from build123d import *

# Parameters (mm, degrees)
F1_DEPTH = 6.35
F2_W     = 4.6636089683
F2_H     = 11.6590159014
F2_H_2   = 4.0806564502
F2_W_2   = 10.2016367018
F2_W_3   = 10.7845924795
F2_H_3   = 15.7396723516
F3_DEPTH = 6.35
F4_W     = 5.2465572953
F4_H     = 11.0760659445
F4_H_2   = 4.0806552861
F4_W_2   = 11.076066643
F4_W_3   = 10.4931145906
F4_H_3   = 15.1567212306
F5_DEPTH = 6.35


with BuildPart() as f1:
    # F0 (on Top) → F1 (new body)
    with BuildSketch(Plane.XY):
        Polygon((72.8688538074, 28.418853879), (-66.7478665709, 28.418853879), (-66.7478665709, -67.4765557051), (-11.9504919276, -67.4765557051), (-11.9504919276, -25.212623179), (15.7396737486, -25.212623179), (15.7396737486, -67.4765557051), (72.8688538074, -67.4765557051), align=None)
        Polygon((-50.1337721944, 0), (-50.1337721944, 15.0109836832), (-37.7460662276, 15.0109836832), (-25.3583602607, 15.0109836832), (-25.3583602607, 0), (-25.3583602607, -15.0109836832), (-37.7460662276, -15.0109836832), (-50.1337721944, -15.0109836832), align=None, mode=Mode.SUBTRACT)
        Polygon((35.2685265243, 0), (35.2685265243, 15.0109836832), (46.7818062752, 15.0109836832), (58.2950860262, 15.0109836832), (58.2950860262, 0), (58.2950860262, -15.0109836832), (46.7818062752, -15.0109836832), (35.2685265243, -15.0109836832), align=None, mode=Mode.SUBTRACT)
        Polygon((0, 76.5122994781), (-66.7478665709, 28.418853879), (72.8688538074, 28.418853879), align=None)
    extrude(amount=F1_DEPTH)

    # F2 (on Top) → F3 (join)
    with BuildSketch(Plane.XY):
        with Locations((46.0531152785, 9.7644259222)):
            Rectangle(F2_W, F2_H)
        with Locations((46.0531152785, 1.8945897464)):
            Rectangle(F2_W, F2_H_2)
        with Locations((38.6204924434, 1.8945897464)):
            Rectangle(F2_W_2, F2_H_2)
        with Locations((53.7772160023, 1.8945897464)):
            Rectangle(F2_W_3, F2_H_2)
        with Locations((46.0531152785, -8.0155746546)):
            Rectangle(F2_W, F2_H_3)
    extrude(amount=F3_DEPTH)

    # F4 (on Top) → F5 (join)
    with BuildSketch(Plane.XY):
        with Locations((-38.1832793355, 9.1814756161)):
            Rectangle(F4_W, F4_H)
        with Locations((-38.1832793355, 1.6031150008)):
            Rectangle(F4_W, F4_H_2)
        with Locations((-46.3445913047, 1.6031150008)):
            Rectangle(F4_W_2, F4_H_2)
        with Locations((-30.3134433925, 1.6031150008)):
            Rectangle(F4_W_3, F4_H_2)
        with Locations((-38.1832793355, -8.0155732576)):
            Rectangle(F4_W, F4_H_3)
    extrude(amount=F5_DEPTH)


solid = f1.part
Source: CAD feature listing. Evaluate the final solid. Frame: model axes, mm. A direction names the side the tool comes from. Round coordinates to 2 decimals unless told otherwise and drop trailing zeros. Order: outer loops, then holes, each group sorted by start corner. A loop starts at its lowest first (then second) coordinate and runs counter-clockwise, first axis right, second up. Notation, with made-up numbers: (61, 19) -> (98, 19) arc R32 ccw to (98, 50) -> close; hole circle Ø5 at (52, 28.5). An arc over 180 degrees is marked (long way). Answer as CSV lines item,"result".
Item 1: Section C-C, the plane y = -12. Return loops of the section in (x, z), plus the area to 3 significant figures.
A:
outline,"(-66.75, 0) -> (-50.13, 0) -> (-50.13, 6.35) -> (-66.75, 6.35) -> close; (-40.81, 0) -> (-35.56, 0) -> (-35.56, 6.35) -> (-40.81, 6.35) -> close; (-25.36, 0) -> (35.27, 0) -> (35.27, 6.35) -> (-25.36, 6.35) -> close; (43.72, 0) -> (48.38, 0) -> (48.38, 6.35) -> (43.72, 6.35) -> close; (58.3, 0) -> (72.87, 0) -> (72.87, 6.35) -> (58.3, 6.35) -> close"
area,"646 mm²"
Item 2: Section B-B, the plane x = 55.5. Return loops of the section in (y, z).
A:
outline,"(-67.48, 0) -> (-15.01, 0) -> (-15.01, 6.35) -> (-67.48, 6.35) -> close; (-0.15, 0) -> (3.93, 0) -> (3.93, 6.35) -> (-0.15, 6.35) -> close; (15.01, 0) -> (39.88, 0) -> (39.88, 6.35) -> (15.01, 6.35) -> close"
Item 3: Pin query (flat end, axial travel): pin 1 Ø1 at (y, z) = (43.5, 3) entering from -X; pin 2 Ø1 at (x, z) = (50.5, 4) entering from +Y. Return the tip coordinate at first contact, or that it passes through.
A:
pin 1,"x = -46.51"
pin 2,"y = 43.51"
Item 4: Reachability of faces 1 (the face through (39, 3.935, 3)), 2 (the face through (72.869, -20, 3)) from +Z, -Z, +X, -X, +Y, -Y: full face, straight path, thin tool, end or side. Return the list, or none.
A:
face 1,"+Z, -Z"
face 2,"+Z, -Z, +X, +Y, -Y"
Item 5: Line query: L1, parallel to X at y = 9, z = 6; L2, parallel to X at y = -37.5, z = 2; L3, parallel to Y at x = 41, z = 2.5. Output: solid intervals per line, ascending.
A:
L1,"-66.75 to -50.13, -40.81 to -35.56, -25.36 to 35.27, 43.72 to 48.38, 58.3 to 72.87"
L2,"-66.75 to -11.95, 15.74 to 72.87"
L3,"-67.48 to -15.01, -0.15 to 3.93, 15.01 to 49.45"
Item 6: Section A-A, the plane y = -27.5. Return loops of the section in (x, z), plus the area to 3 significant figures.
A:
outline,"(-66.75, 0) -> (-11.95, 0) -> (-11.95, 6.35) -> (-66.75, 6.35) -> close; (15.74, 0) -> (72.87, 0) -> (72.87, 6.35) -> (15.74, 6.35) -> close"
area,"711 mm²"
Item 7: Pull-direction query (Y, two-part tool) for faces 3 (the face through (-11.95, -47, 3)), 4 (the face through (58.295, -7, 3)); classes: pulls with the +Y half, pulls with the -Y half, needs draft (parallel to the pull), parting line crosses it, or undercut.
A:
face 3,"needs draft"
face 4,"undercut"
Item 8: Section D-D, the plane z = 4. Count the separate pieces of the cut face and the enclosed holes in it, plus the area to 3 significant figures.
A:
separate pieces,"1"
enclosed holes,"7"
area,"14,600 mm²"
